Read the model definition and answer for the solid it produces. Units are mm, in the model's axes. A direction names the side the tool comes from. Round coordinates to 2 decimals unless told otherwise and drop trailing zeros. Order: outer loops, then holes, each group sorted by start corner. A loop starts at its lowest first (then second) coordinate and runs counter-clockwise, first axis right, second up. Notation, with made-up numbers: M 64.25,-12 L 108.25,-12 A23 ccw 108.25,3 Z; hole C 69,85.25 d6. An arc over 180 degrees is marked long. Use one line per item in the form item = value. Start each with the question number.
from build123d import *
from OCP.BRepAlgoAPI import BRepAlgoAPI_Cut
from OCP.TopTools import TopTools_ListOfShape


with BuildPart() as part:
    # 草图1 → 旋转1 (revolve)
    with BuildSketch(Plane.XY):
        Polygon((2.3, 0), (2.3, 0.9), (0, 0.9), (0, 4.5), (3.15, 4.5), (3.15, 1), (3.75, 1), (3.75, 0), align=None)
    revolve(axis=Axis((0, 0.9, 0), (0, 1, 0)))


with BuildPart() as cut_revolve_6_tool:
    # 草图2 → 切除-旋转6 (revolve)
    with BuildSketch(Plane.XY):
        with BuildLine():
            Line((1.45, 4.5), (3.15, 4.5))
            Line((3.15, 4.5), (3.15, 3.8))
            add(Edge.make_bspline(
                [(1.45, 4.5), (2.373616695, 4.5), (2.769590277, 4.433977798), (3.153202517, 4.267640833), (3.15, 4.025903219), (3.15, 3.8)],
                knots=[0, 0, 0, 0, 0.535445213, 0.635445213, 1, 1, 1, 1], degree=3))
        make_face()
    revolve(axis=Axis((0, 4.5, 0), (0, -1, 0)))


with BuildPart() as part_1:
    add(part.part)

    # 切除-旋转6: cut by cut_revolve_6_tool, with a tolerance
    cut_revolve_6_stock = TopTools_ListOfShape()
    cut_revolve_6_stock.Append(part_1.part.wrapped)
    cut_revolve_6_tools = TopTools_ListOfShape()
    cut_revolve_6_tools.Append(cut_revolve_6_tool.part.wrapped)
    cut_revolve_6_cut = BRepAlgoAPI_Cut()
    cut_revolve_6_cut.SetArguments(cut_revolve_6_stock)
    cut_revolve_6_cut.SetTools(cut_revolve_6_tools)
    cut_revolve_6_cut.SetFuzzyValue(0.00001)
    cut_revolve_6_cut.Build()
    add(Compound.cast(cut_revolve_6_cut.Shape()).solids(), mode=Mode.REPLACE)


solid = part_1.part
Item 1: A tool of negligible diameter and unlimited length cuts with its end or side. For faces 4 (the flat face through (0, 0.9, 0)), 5 (the cylindrical face through (-2.5, 2.402, 1.917)), 6 (the flat face through (-2, 0, 2)), from which of +Z, -Z, +X, -X, +Y, -Y can it reach the whole face along a straight path? Write none if from no direction.
Item 2: For a pull along X with two mould halves and no side action, classify faces 1 (the cylindrical face through (-1.825, 0.456, 1.4)), 2 (the flat face through (0, 4.5, 0)), 3 (the cylindrical face through (-3.746, 0.493, -0.165)) as pulls with the +X half, pulls with the -X half, needs draft (parallel to the pull), parting line crosses it, or undercut.
Item 3: Find the intervals of material crossed by L1, parallel to Z at x = 0, y = 0.7; L2, parallel to Y at x = 0.75, z = 1.25, in increasing order. Write a range as [from, to].
Item 4: Section B-B (y = 2) is taken. Write down the section's boundary in (x, z), and give its area (3 significant figures).
Item 5: Section A-A (y = 0.5) is taken. Write down the section's boundary in (x, z).
Item 6: Given P1, Ø1, axis at y = 2, z = 1, coming from the +X side, flat-ended and moving along its own axis, determine where the tip first touches the part or whether it passes through.
The answers:
q1.face_4 = -Y
q1.face_5 = +Y
q1.face_6 = +Z, -Z, +X, -X, -Y
q2.face_1 = undercut
q2.face_2 = needs draft
q2.face_3 = parting line crosses it
q3.L1 = [-3.75, -2.3], [2.3, 3.75]
q3.L2 = [0.9, 4.5]
q4.outline = C 0,0 d6.3
q4.area = 31.2 mm²
q5.outline = C 0,0 d7.5; hole C 0,0 d4.6
q6.P1 = 3.11
